```python
from build123d import *

# Parameters (mm, degrees)
SKETCH_1_R           = 17.9
EXTRUDE_1_DEPTH      = 53.5
SKETCH_2_R           = 6.5
EXTRUDE_2_DEPTH      = 4.5
SKETCH_2_3_R         = 1.5
CUT_EXTRUDE_1_DEPTH  = 10
SKETCH_5_R           = 1.585
EXTRUDE_3_DEPTH      = 9
CUT_EXTRUDE_START    = -1.5
SKETCH_5_3_R         = 5
SKETCH_5_3_R_2       = 1.585
CUT_EXTRUDE_2_DEPTH  = 1.5
CUT_EXTRUDE_3_DEPTH  = 5
SKETCH_8_R           = 16
CUT_EXTRUDE_4_DEPTH  = 48.5
SKETCH_1_5_R         = 7.5
EXTRUDE_5_DEPTH      = 4.5
SKETCH_1_7_R         = 17
SKETCH_1_7_R_2       = 12
SKETCH_1_7_W         = 1
SKETCH_1_7_H         = 5
CUT_EXTRUDE_6_DEPTH  = 2
SKETCH_1_8_W         = 1
SKETCH_1_8_H         = 5
EXTRUDE_6_DEPTH      = 9
FILLET_5_R           = 1
FILLET_9_R           = 1
FILLET_10_R          = 1.5
SKETCH_10_R          = 1
CUT_EXTRUDE_9_DEPTH  = 1
CUT_EXTRUDE_START_2  = -1
SKETCH_11_R          = 1
CUT_EXTRUDE_10_DEPTH = 1
FILLET_11_R          = 1
SKETCH_12_R          = 5.5
CUT_EXTRUDE_11_DEPTH = 2
EXTRUDE_START        = 8
SKETCH_13_R          = 1.585
EXTRUDE_7_DEPTH      = 8
FILLET_20_R          = 0.5


with BuildPart() as part:
    # Эскиз1 → Бобышка-Вытянуть1 (new body)
    with BuildSketch(Plane.XY):
        Circle(SKETCH_1_R)
    extrude(amount=EXTRUDE_1_DEPTH)

    # Эскиз2 → Бобышка-Вытянуть2 (add)
    with BuildSketch(Plane.XY.offset(53.5)):
        Circle(SKETCH_2_R)
    extrude(amount=EXTRUDE_2_DEPTH)

    # Эскиз2<3> → Вырез-Вытянуть1 (cut)
    with BuildSketch(Plane.XY.offset(53.5)):
        with Locations((12.5, 0)):
            Circle(SKETCH_2_3_R)
        with Locations((-12.5, 0)):
            Circle(SKETCH_2_3_R)
    extrude(amount=-CUT_EXTRUDE_1_DEPTH, mode=Mode.SUBTRACT)

    # Эскиз5 → Бобышка-Вытянуть3 (add)
    with BuildSketch(Plane.XY.offset(58)):
        Circle(SKETCH_5_R)
    extrude(amount=EXTRUDE_3_DEPTH)

    # Эскиз5<3> → Вырез-Вытянуть2 (cut)
    with BuildSketch(Plane.XY.offset(58).offset(CUT_EXTRUDE_START)):
        Circle(SKETCH_5_3_R)
        Circle(SKETCH_5_3_R_2, mode=Mode.SUBTRACT)
    extrude(amount=CUT_EXTRUDE_2_DEPTH, mode=Mode.SUBTRACT)

    # Эскиз2<4> → Вырез-Вытянуть3 (cut)
    with BuildSketch(Plane.XY.offset(53.5)):
        with BuildLine():
            ThreePointArc((-3.826834324, 9.238795325), (-7.071067812, 7.071067812), (-9.238795325, 3.826834324))
            ThreePointArc((-9.238795325, 3.826834324), (-11.851921255, 2.744442123), (-12.934313455, 5.357568053))
            ThreePointArc((-12.934313455, 5.357568053), (-9.899494937, 9.899494937), (-5.357568053, 12.934313455))
            ThreePointArc((-5.357568053, 12.934313455), (-2.744442123, 11.851921255), (-3.826834324, 9.238795325))
        make_face()
        with BuildLine():
            ThreePointArc((12.934313455, 5.357568053), (9.899494937, 9.899494937), (5.357568053, 12.934313455))
            ThreePointArc((5.357568053, 12.934313455), (2.744442123, 11.851921255), (3.826834324, 9.238795325))
            ThreePointArc((3.826834324, 9.238795325), (7.071067812, 7.071067812), (9.238795325, 3.826834324))
            ThreePointArc((9.238795325, 3.826834324), (11.851921255, 2.744442123), (12.934313455, 5.357568053))
        make_face()
        with BuildLine():
            ThreePointArc((12.934313455, -5.357568053), (11.851921255, -2.744442123), (9.238795325, -3.826834324))
            ThreePointArc((9.238795325, -3.826834324), (7.071067812, -7.071067812), (3.826834324, -9.238795325))
            ThreePointArc((3.826834324, -9.238795325), (2.744442123, -11.851921255), (5.357568053, -12.934313455))
            ThreePointArc((5.357568053, -12.934313455), (9.899494937, -9.899494937), (12.934313455, -5.357568053))
        make_face()
        with BuildLine():
            ThreePointArc((-5.357568053, -12.934313455), (-2.744442123, -11.851921255), (-3.826834324, -9.238795325))
            ThreePointArc((-3.826834324, -9.238795325), (-7.071067812, -7.071067812), (-9.238795325, -3.826834324))
            ThreePointArc((-9.238795325, -3.826834324), (-11.851921255, -2.744442123), (-12.934313455, -5.357568053))
            ThreePointArc((-12.934313455, -5.357568053), (-9.899494937, -9.899494937), (-5.357568053, -12.934313455))
        make_face()
    extrude(amount=-CUT_EXTRUDE_3_DEPTH, mode=Mode.SUBTRACT)

    # Эскиз8 → Вырез-Вытянуть4 (cut)
    with BuildSketch(Plane.XY.offset(3)):
        with Locations(Location((0, 0, 0), (0, 0, 180))):
            Circle(SKETCH_8_R)
    extrude(amount=CUT_EXTRUDE_4_DEPTH, mode=Mode.SUBTRACT)

    # Эскиз1<5> → Бобышка-Вытянуть5 (add)
    with BuildSketch(Plane.XY):
        Circle(SKETCH_1_5_R)
    extrude(amount=-EXTRUDE_5_DEPTH)

    # Эскиз1<7> → Вырез-Вытянуть6 (cut)
    with BuildSketch(Plane.XY):
        Circle(SKETCH_1_7_R)
        Circle(SKETCH_1_7_R_2, mode=Mode.SUBTRACT)
        with Locations((-14.5, 0)):
            Rectangle(SKETCH_1_7_W, SKETCH_1_7_H, mode=Mode.SUBTRACT)
        with Locations((14.5, 0)):
            Rectangle(SKETCH_1_7_W, SKETCH_1_7_H, mode=Mode.SUBTRACT)
    extrude(amount=CUT_EXTRUDE_6_DEPTH, mode=Mode.SUBTRACT)

    # Эскиз1<8> → Бобышка-Вытянуть6 (add)
    with BuildSketch(Plane.XY):
        with Locations((14.5, 0)):
            Rectangle(SKETCH_1_8_W, SKETCH_1_8_H)
        with Locations((-14.5, 0)):
            Rectangle(SKETCH_1_8_W, SKETCH_1_8_H)
    extrude(amount=-EXTRUDE_6_DEPTH)

    # Скругление5
    fillet_5_edges = [part.edges().sort_by_distance(p)[0] for p in [
        (-12, 0, 0),
    ]]
    fillet(fillet_5_edges, radius=FILLET_5_R)

    # Скругление9
    fillet_9_edges = [part.edges().sort_by_distance(p)[0] for p in [
        (-7.5, 0, -4.5),
    ]]
    fillet(fillet_9_edges, radius=FILLET_9_R)

    # Скругление10
    fillet_10_edges = [part.edges().sort_by_distance(p)[0] for p in [
        (-17.9, 0, 53.5),
    ]]
    fillet(fillet_10_edges, radius=FILLET_10_R)

    # Эскиз10 → Вырез-Вытянуть9 (cut)
    with BuildSketch(Plane(origin=(15, 0, 0), x_dir=(0, 0, -1), z_dir=(1, 0, 0))):
        with Locations(Location((6.5, 0, 0), (0, 0, 90))):
            Circle(SKETCH_10_R)
    extrude(amount=-CUT_EXTRUDE_9_DEPTH, mode=Mode.SUBTRACT)

    # Эскиз11 → Вырез-Вытянуть10 (cut)
    with BuildSketch(Plane.ZY.offset(15).offset(CUT_EXTRUDE_START_2)):
        with Locations(Location((-6.5, 0, 0), (0, 0, 90))):
            Circle(SKETCH_11_R)
    extrude(amount=CUT_EXTRUDE_10_DEPTH, mode=Mode.SUBTRACT)

    # Скругление11
    fillet_11_edges = [part.edges().sort_by_distance(p)[0] for p in [
        (-14.5, -2.5, -9),
        (-14.5, 2.5, -9),
        (14.5, 2.5, -9),
        (14.5, -2.5, -9),
    ]]
    fillet(fillet_11_edges, radius=FILLET_11_R)

    # Эскиз12 → Вырез-Вытянуть11 (cut)
    with BuildSketch(Plane(origin=(0, 0, -4.5), x_dir=(-1, 0, 0), z_dir=(0, 0, -1))):
        Circle(SKETCH_12_R)
    extrude(amount=-CUT_EXTRUDE_11_DEPTH, mode=Mode.SUBTRACT)

    # Эскиз13 → Бобышка-Вытянуть7 (add)
    with BuildSketch(Plane(origin=(0, 0, -2.5), x_dir=(-1, 0, 0), z_dir=(0, 0, -1)).offset(EXTRUDE_START)):
        with Locations(Location((0, 0, 0), (0, 0, 180))):
            Circle(SKETCH_13_R)
    extrude(amount=-EXTRUDE_7_DEPTH)

    # Скругление20
    fillet_20_edges = [part.edges().sort_by_distance(p)[0] for p in [
        (-1.585, 0, -10.5),
    ]]
    fillet(fillet_20_edges, radius=FILLET_20_R)


solid = part.part
```
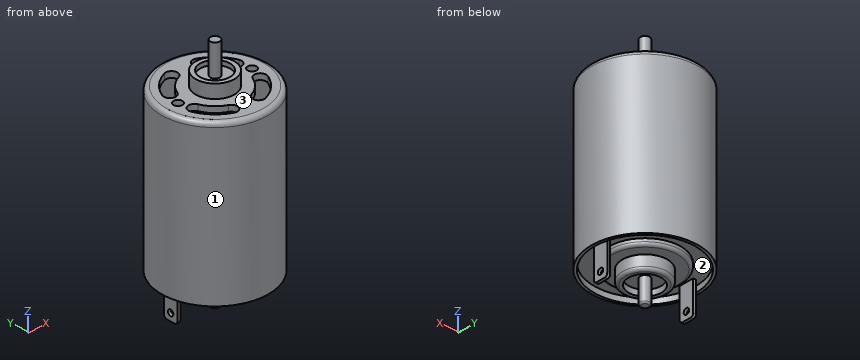
Geometry check sheet. Reference: the model listing, model coordinates, mm. Face numbers are marked on the shaded views. Coordinates: 2 decimals unless noted, no trailing zeros. Order: outer loops, then holes, each group sorted by start corner. A loop starts at its lowest first (then second) coordinate and runs counter-clockwise, first axis right, second up.
Item 1: Section check A-A (z = -6.5). Enter the section's corners in (x, y) (3 decimals), plus the area to 3 significant figures.
Item 2: Scan lines: line 1 along Y through (x, z) = (0, 1.4); line 2 along Y through (x, z) = (-0.5, 15); line 3 along Z through (x, y) = (-3, 15). Record each from-to range of solid material in increasing order.
Item 3: Section check B-B (z = 46.5). Enter the section's corners in (x, y).
Item 4: Mould release check, pull along Y, two halves, no side actions. Record for the marked faces 1, 2 and 3: released by +Y, released by -Y, zero draft, split by the parting line, or undercut.
Item 5: Depth check by flat-ended pin: pin 1 (12 mm diameter, centred on x = 3, z = 49.5, fed in from +Y); pin 2 (3 mm diameter, centred on y = 8.5, z = 29.5, fed in from +X); pin 3 (2 mm diameter, centred on x = 13.5, z = 49.5, fed in from +Y); pin 4 (8 mm diameter, centred on y = 12, z = 59, fed in from -X). Enter the tip coordinate at first touch or a pass-through.
Check sheet entries:
1. outline: (-15, -2.5) - (-14, -2.5) - (-14, -1) - (-15, -1) - close; (-15, 1) - (-14, 1) - (-14, 2.5) - (-15, 2.5) - close; circle Ø3.17 at (0, 0); (14, -2.5) - (15, -2.5) - (15, -1) - (14, -1) - close; (14, 1) - (15, 1) - (15, 2.5) - (14, 2.5) - close
1. area: 13.9 mm2
2. line 1: y = -17.9 to -17, -12 to 12, 17 to 17.9
2. line 2: y = -17.89 to -15.99, 15.99 to 17.89
2. line 3: z = 2 to 3, 51.5 to 53.5
3. outline: circle Ø35.8 at (0, 0); hole circle Ø32 at (0, 0)
4. face 1: split by the parting line
4. face 2: undercut
4. face 3: zero draft
5. pin 1: stops at y = 17.9
5. pin 2: stops at x = 16.47
5. pin 3: stops at y = 12.81
5. pin 4: passes through
